For this review, take the finished solid that the model builds, in its own axes (mm). A direction names the side the tool comes from. Coordinates: 2 decimals unless noted, no trailing zeros. Write each loop counter-clockwise with the first axis right and the second up, starting at its lowest first coordinate (ties: lowest second). Pieces come first, ordered by that corner, then holes. Notation, with made-up numbers: (7, -38.75) -> (48, -38.75) arc R34 cw to (48, 0.25) -> close; hole circle Ø10 at (5.5, 39). An arc over 180 degrees is marked (long way). Put each result on its own line as item: value. Start each with the question number.
Item 1: To check wall thickness, follow L1, parallel to Y at x = 0, z = 3.2; L2, parallel to X at y = 28.5, z = 4.2; L3, parallel to X at y = 46, z = 2.9. State the ranges of each line that lie inside material, in increasing order.
Item 2: Consider section A-A on y = 9.5. Give the boundary of the cut face in (x, z), and give its area (3 significant figures).
Item 3: For faces 5 (the conical face through (10.92, 20.34, 0.13)), 6 (the flat face through (-38.683, 45.033, 0.127)), 7 (the flat face through (26.035, 33.8, 4.377)), 8 (the conical face through (68.486, 18.465, 4.377)), 9 (the flat face through (-27, 19, 2)), list the 3-axis set-ups (+Z, -Z, +X, -X, +Y, -Y) from which the entire face can be reached by the end or side of a thin tool; tool diameter is ignored.
Item 4: Insertion check: P1, Ø1.5, axis at y = 52, z = 2.5, coming from the -X side; P2, Ø4.5, axis at x = -60, y = 9.5, coming from the -Z side; P3, Ø2, axis at y = 31.5, z = 2.5, coming from the +X side; P4, Ø1.2, axis at y = 35, z = 1.5, coming from the -X side. Each pin has a flat end and moves straight along its axis. Give the tip position at first contact, or say it passes through.
Item 5: Consider section C-C on x = 0. Give the boundary of the cut face in (y, z), and give its area (3 significant figures).
Item 6: The part is to be moulded in two halves that separate along Y. For faces 1 (the flat face through (28, 19, 2)), 2 (the conical face through (-9.18, 69.28, 4.38)), 3 (the flat face through (-1, 20, 0)), 4 (the conical face through (10.915, 20.335, 4.377)), say which applies: +Y half, -Y half, draft (parallel to the pull), parting line (faces both ways), or undercut.
Item 7: Consider section D-D on y = 29. Give the number of separate pieces and of enclosed holes in the cut face, and give its area (3 significant figures).
Item 8: Consider section B-B on z = 3.1. Give the boundary of the cut face in (x, y).
```python
from build123d import *

# Parameters (mm, degrees)
F1_DEPTH = 4.5
F2_R     = 2.75
F3_DEPTH = 4.501
F4_R     = 5
F5_R     = 1
F6_R     = 10
F7_R     = 2
F8_SIZE  = 0.25


with BuildPart() as f1:
    # F0 (on Top) → F1 (new body)
    with BuildSketch(Plane.XY):
        Polygon((-9.5, 70), (-69.5, 19), (-69.5, 0), (69.5, 0), (69.5, 19), (9.5, 70), align=None)
        Polygon((-43.2511905032, 19), (-9.5, 47.6885119277), (-9.5, 19), align=None, mode=Mode.SUBTRACT)
        Polygon((9.5, 19), (9.5, 47.6885119277), (43.2511905032, 19), align=None, mode=Mode.SUBTRACT)
    extrude(amount=F1_DEPTH)

    # F2 (on face) → F3 (cut, through all)
    with BuildSketch(Plane.XY.offset(4.5)):
        with Locations((0, 60.5)):
            Circle(F2_R)
        with Locations((0, 29)):
            Circle(F2_R)
        with Locations((60, 9.5)):
            Circle(F2_R)
        with Locations((-60, 9.5)):
            Circle(F2_R)
    extrude(amount=-F3_DEPTH, mode=Mode.SUBTRACT)

    # F4
    f4_edges = [f1.edges().sort_by_distance(p)[0] for p in [
        (-9.5, 19, 2.25),
        (9.5, 19, 2.25),
    ]]
    fillet(f4_edges, radius=F4_R)

    # F5
    f5_edges = [f1.edges().sort_by_distance(p)[0] for p in [
        (43.251191, 19, 2.25),
        (9.5, 47.688512, 2.25),
        (-9.5, 47.688512, 2.25),
        (-43.251191, 19, 2.25),
    ]]
    fillet(f5_edges, radius=F5_R)

    # F6
    f6_edges = [f1.edges().sort_by_distance(p)[0] for p in [
        (-9.5, 70, 2.25),
        (9.5, 70, 2.25),
        (-69.5, 19, 2.25),
        (69.5, 19, 2.25),
    ]]
    fillet(f6_edges, radius=F6_R)

    # F7
    f7_edges = [f1.edges().sort_by_distance(p)[0] for p in [
        (-69.5, 0, 2.25),
        (69.5, 0, 2.25),
    ]]
    fillet(f7_edges, radius=F7_R)

    # F8
    f8_edges = [f1.edges().sort_by_distance(p)[0] for p in [
        (-2.75, 60.5, 4.5),
        (-2.75, 29, 4.5),
        (57.25, 9.5, 4.5),
        (-62.75, 9.5, 4.5),
        (-2.75, 60.5, 0),
        (-62.75, 9.5, 0),
        (-2.75, 29, 0),
        (57.25, 9.5, 0),
        (0, 0, 4.5),
        (0, 0, 0),
        (-27.515336, 19, 0),
        (-69.5, 8.187798, 4.5),
        (-68.914214, 0.585786, 4.5),
        (-68.576476, 18.572925, 4.5),
        (-39.138599, 44.807191, 4.5),
        (68.914214, 0.585786, 4.5),
        (-9.274307, 69.385998, 4.5),
        (69.5, 8.187798, 4.5),
        (0, 70, 4.5),
        (68.576476, 18.572925, 4.5),
        (9.274307, 69.385998, 4.5),
        (39.138599, 44.807191, 4.5),
        (-27.515336, 19, 4.5),
        (-41.469272, 19.654992, 4.5),
        (-10.964466, 20.464466, 4.5),
        (-26.162985, 33.524975, 4.5),
        (-9.5, 34.763036, 4.5),
        (-10.080267, 46.433719, 4.5),
        (9.5, 34.763036, 4.5),
        (10.080267, 46.433719, 4.5),
        (10.964466, 20.464466, 4.5),
        (26.162985, 33.524975, 4.5),
        (27.515336, 19, 4.5),
        (41.469272, 19.654992, 4.5),
        (-69.5, 8.187798, 0),
        (-68.914214, 0.585786, 0),
        (-68.576476, 18.572925, 0),
        (-39.138599, 44.807191, 0),
        (68.914214, 0.585786, 0),
        (-9.274307, 69.385998, 0),
        (69.5, 8.187798, 0),
        (0, 70, 0),
        (68.576476, 18.572925, 0),
        (9.274307, 69.385998, 0),
        (39.138599, 44.807191, 0),
        (-41.469272, 19.654992, 0),
        (-10.964466, 20.464466, 0),
        (-26.162985, 33.524975, 0),
        (-9.5, 34.763036, 0),
        (-10.080267, 46.433719, 0),
        (9.5, 34.763036, 0),
        (10.080267, 46.433719, 0),
        (10.964466, 20.464466, 0),
        (26.162985, 33.524975, 0),
        (27.515336, 19, 0),
        (41.469272, 19.654992, 0),
    ]]
    chamfer(f8_edges, length=F8_SIZE)


solid = f1.part
```
Return value:
1. L1: 0 to 26.25, 31.75 to 57.75, 63.25 to 70
1. L2: -58.32 to -32.07, -9.5 to -2.7, 2.7 to 9.5, 32.07 to 58.32
1. L3: -37.74 to -11.49, -9.62 to 9.62, 11.49 to 37.74
2. outline: (-69.5, 0.25) -> (-69.25, 0) -> (-63, 0) -> (-62.75, 0.25) -> (-62.75, 4.25) -> (-63, 4.5) -> (-69.25, 4.5) -> (-69.5, 4.25) -> close; (-57.25, 0.25) -> (-57, 0) -> (57, 0) -> (57.25, 0.25) -> (57.25, 4.25) -> (57, 4.5) -> (-57, 4.5) -> (-57.25, 4.25) -> close; (62.75, 0.25) -> (63, 0) -> (69.25, 0) -> (69.5, 0.25) -> (69.5, 4.25) -> (69.25, 4.5) -> (63, 4.5) -> (62.75, 4.25) -> close
2. area: 576 mm^2
3. face 5: -Z
3. face 6: -Z, -X, +Y
3. face 7: +Z
3. face 8: +Z, +X, +Y
3. face 9: +Z, -Z
4. P1: x = -31.56
4. P2: through
4. P3: x = 55.97
4. P4: x = -51.38
5. outline: (0, 0.25) -> (0.25, 0) -> (26, 0) -> (26.25, 0.25) -> (26.25, 4.25) -> (26, 4.5) -> (0.25, 4.5) -> (0, 4.25) -> close; (31.75, 0.25) -> (32, 0) -> (57.5, 0) -> (57.75, 0.25) -> (57.75, 4.25) -> (57.5, 4.5) -> (32, 4.5) -> (31.75, 4.25) -> close; (63.25, 0.25) -> (63.5, 0) -> (69.75, 0) -> (70, 0.25) -> (70, 4.25) -> (69.75, 4.5) -> (63.5, 4.5) -> (63.25, 4.25) -> close
5. area: 265 mm^2
6. face 1: undercut
6. face 2: +Y half
6. face 3: draft
6. face 4: undercut
7. separate pieces: 4
7. enclosed holes: 0
7. area: 296 mm^2
8. outline: (-69.5, 2) arc R2 ccw to (-67.5, 0) -> (67.5, 0) arc R2 ccw to (69.5, 2) -> (69.5, 14.38) arc R10 ccw to (65.98, 21.99) -> (12.3, 67.62) arc R10 ccw to (5.82, 70) -> (-5.82, 70) arc R10 ccw to (-12.3, 67.62) -> (-65.98, 21.99) arc R10 ccw to (-69.5, 14.38) -> close; hole circle Ø5.5 at (-60, 9.5); hole (-41.18, 20.76) arc R1 ccw to (-40.53, 19) -> (-14.5, 19) arc R5 ccw to (-9.5, 24) -> (-9.5, 45.53) arc R1 ccw to (-11.15, 46.29) -> close; hole circle Ø5.5 at (0, 29); hole circle Ø5.5 at (0, 60.5); hole (9.5, 24) arc R5 ccw to (14.5, 19) -> (40.53, 19) arc R1 ccw to (41.18, 20.76) -> (11.15, 46.29) arc R1 ccw to (9.5, 45.53) -> close; hole circle Ø5.5 at (60, 9.5)
